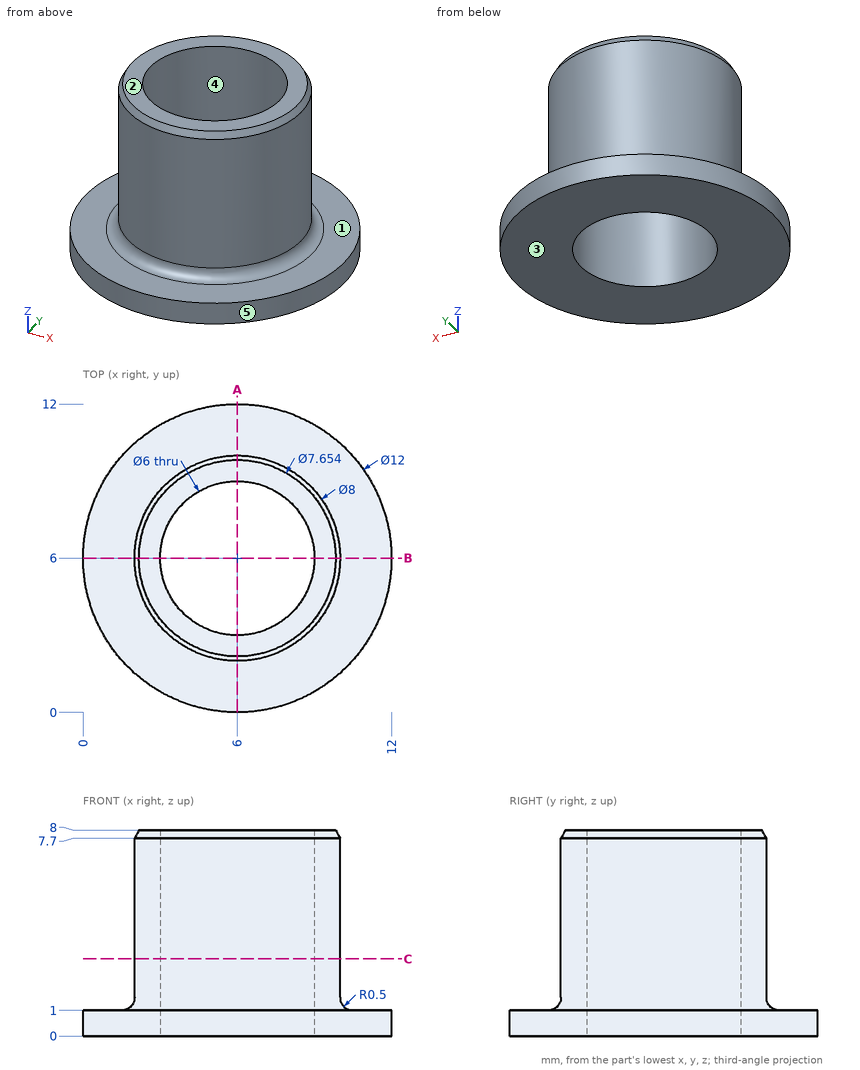
For this review, use the dimensioned drawing (mm, ordinates from the lowest corner) and the shaded views. A direction names the side the tool comes from. Give positions to 0.01 mm unless a question says otherwise; leave off trailing zeros. Order: outer loops, then holes, each group sorted by start corner. A loop starts at its lowest first (then second) coordinate and runs counter-clockwise, first axis right, second up.
1) Insertion check: pin 1 (1.5 mm diameter, centred on y = 3, z = 6.5, fed in from +X); pin 2 (3 mm diameter, centred on y = 3.5, z = 5, fed in from -X); pin 3 (3 mm diameter, centred on y = 5, z = 6, fed in from +X). Each pin has a flat end and moves straight along its axis. Give the tip position at first contact, or say it passes through.
2) Wall thickness on line 1 (X direction, y = 6, z = 3); line 2 (Z direction, x = 10.75, y = 7); line 3 (Y direction, x = 5.5, z = 2): over which ranges is each line inside the solid? List them lowest first.
3) Take a section at C-C (z = 3). Give the boundary of the cut face in (x, y).
4) For the marked faces 1 and 2, list the 3-axis set-ups (+Z, -Z, +X, -X, +Y, -Y) from which the entire face can be reached by the end or side of a thin tool; tool diameter is ignored.
5) The part is to be moulded in two halves that separate along X. For the marked faces 3, 4 and 5, say which applies: released by +X, released by -X, zero draft, split by the parting line, or undercut.
6) Take a section at A-A (x = 6). Give the boundary of the cut face in (y, z).
Derived:
1. pin 1: stops at x = 9.31
1. pin 2: stops at x = 2.13
1. pin 3: stops at x = 10
2. line 1: x = 2 to 3, 9 to 10
2. line 2: z = 0 to 1
2. line 3: y = 2.03 to 3.04, 8.96 to 9.97
3. outline: circle Ø8 at (6, 6); hole circle Ø6 at (6, 6)
4. face 1: +Z
4. face 2: +Z, +X, -X, +Y, -Y
5. face 3: zero draft
5. face 4: undercut
5. face 5: split by the parting line
6. outline: (0, 0) - (3, 0) - (3, 8) - (2.17, 8) - (2, 7.7) - (2, 1.5) arc R0.5 cw to (1.5, 1) - (0, 1) - close; (9, 0) - (12, 0) - (12, 1) - (10.5, 1) arc R0.5 cw to (10, 1.5) - (10, 7.7) - (9.83, 8) - (9, 8) - close
